```python
from build123d import *

# Parameters (mm, degrees)
SKETCH1_R                = 7.5
SKETCH1_R_2              = 3.15
BOSS_EXTRUDE1_DEPTH      = 13
BOSS_EXTRUDE2_START      = 10
SKETCH2_R                = 7.5
BOSS_EXTRUDE2_DEPTH      = 10
BOSS_EXTRUDE4_DEPTH      = 5
BOSS_EXTRUDE4_DEPTH_BACK = 10
SKETCH7_R                = 4.7
CUT_EXTRUDE2_DEPTH       = 20
SKETCH9_R                = 2.2
CUT_EXTRUDE4_DEPTH       = 37.626493144
CUT_EXTRUDE5_REACH       = 33.329
CUT_EXTRUDE5_END_RADIUS  = 7.5
SKETCH4_R                = 2.5


with BuildPart() as part:
    # Sketch1 → Boss-Extrude1 (new body)
    with BuildSketch(Plane(origin=(0, 0, 0), x_dir=(1, 0, 0), z_dir=(0, 1, 0))):
        with Locations(Location((0, 0, 0), (0, 0, 90))):
            Circle(SKETCH1_R)
        with Locations(Location((0, 0, 0), (0, 0, 90))):
            Circle(SKETCH1_R_2, mode=Mode.SUBTRACT)
    extrude(amount=BOSS_EXTRUDE1_DEPTH)

    # Sketch2 → Boss-Extrude2 (add)
    with BuildSketch(Plane.XZ.offset(BOSS_EXTRUDE2_START)):
        with Locations(Location((0, 0, 0), (0, 0, 270))):
            Circle(SKETCH2_R)
    extrude(amount=-BOSS_EXTRUDE2_DEPTH)

    # Sketch6 → Boss-Extrude4 (add, two sides: drawn at the far end of the back side and taken through both)
    with BuildSketch(Plane(origin=(0, 0, 0), x_dir=(1, 0, 0), z_dir=(0, 1, 0)).offset(-BOSS_EXTRUDE4_DEPTH_BACK)):
        with BuildLine():
            Line((-7.5, 0), (-7.5, 27.5))
            Line((-7.5, 27.5), (7.5, 27.5))
            Line((7.5, 27.5), (7.5, 0))
            ThreePointArc((7.5, 0), (0, 7.5), (-7.5, 0))
        make_face()
    extrude(amount=BOSS_EXTRUDE4_DEPTH + BOSS_EXTRUDE4_DEPTH_BACK)

    # Sketch7 → Cut-Extrude2 (cut)
    with BuildSketch(Plane(origin=(0, 0, -27.5), x_dir=(-1, 0, 0), z_dir=(0, 0, -1))):
        with Locations((0, -2.5)):
            Circle(SKETCH7_R)
    extrude(amount=-CUT_EXTRUDE2_DEPTH, mode=Mode.SUBTRACT)

    # Sketch9 → Cut-Extrude4 (cut, through all)
    with BuildSketch(Plane.XZ.offset(10)):
        with Locations(Location((0, -20.5, 0), (0, 0, 270))):
            Circle(SKETCH9_R)
    extrude(amount=-CUT_EXTRUDE4_DEPTH, mode=Mode.SUBTRACT)

    # Cut-Extrude5: up to this cylinder (the profile starts inside it)
    cut_extrude5_end = Plane(origin=(0, 7.53728, 0), z_dir=(0, -1, 0)) * Cylinder(CUT_EXTRUDE5_END_RADIUS, 82.658, mode=Mode.PRIVATE)
    # Sketch4 → Cut-Extrude5 (cut, up to the surface)
    with BuildSketch(Plane.XY, mode=Mode.PRIVATE) as cut_extrude5_sk1:
        with Locations(Location((0, 7.537279813, 0), (0, 0, 180))):
            Circle(SKETCH4_R)
    cut_extrude5_tool1 = extrude(cut_extrude5_sk1.sketch, amount=CUT_EXTRUDE5_REACH, mode=Mode.PRIVATE) & cut_extrude5_end
    add(cut_extrude5_tool1.solids().sort_by_distance((0, 7.53728, 0))[0], mode=Mode.SUBTRACT)


solid = part.part
```
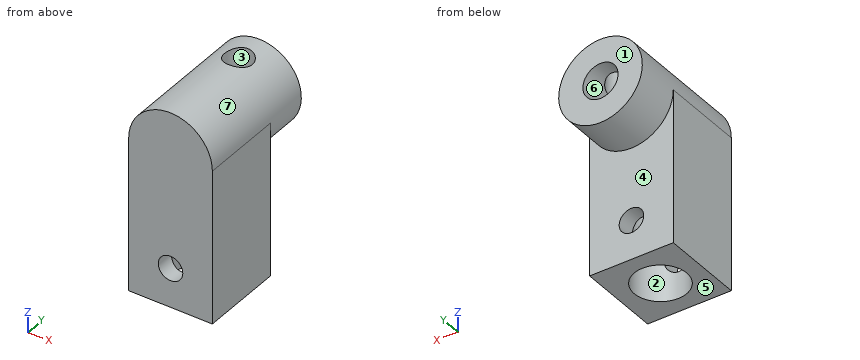
Can you work these out from the model? Positions are in its coordinate system, mm. Face numbers are marked on the shaded views. A direction names the side the tool comes from. Coordinates: 2 decimals unless noted, no trailing zeros. Loops run counter-clockwise (first coordinate to the right, second up) from the corner with the lowest first, then second, coordinate; pieces in that order, holes last. Notation, with made-up numbers: (62, 82.25) - (103, 82.25) arc R18 cw to (103, 106.25) - close; hole circle Ø2 at (82.25, 19). An arc over 180 degrees is marked (long way). Use a Markdown table: item, result.
Item 1: Will these pins go through, and if not, where does the flat tip stop? pin 1 (4 mm diameter, centred on x = 0, z = -20.5, fed in from +Y); pin 2 (3 mm diameter, centred on x = -3.5, y = -5.5, fed in from +Z); pin 3 (6 mm diameter, centred on x = 1.5, z = 1.5, fed in from +Y); pin 4 (4 mm diameter, centred on x = 0, z = 0, fed in from +Y).
Numbers:
| item | result |
|---|---|
| pin 1 | passes through |
| pin 2 | stops at z = 7.23 |
| pin 3 | stops at y = 13 |
| pin 4 | stops at y = 0 |
Item 2: I want a section at A-A on z = -20.5. Please give me the cut outline in (x, y).
Numbers:
| item | result |
|---|---|
| outline | (-7.5, -10) - (-2.2, -10) - (-2.2, -6.65) arc R4.7 cw to (-2.2, 1.65) - (-2.2, 5) - (-7.5, 5) - close; (2.2, -10) - (7.5, -10) - (7.5, 5) - (2.2, 5) - (2.2, 1.65) arc R4.7 cw to (2.2, -6.65) - close |
Item 3: I want a section at D-D on z = -13. Please give me the cut outline in (x, y), and give its area (3 significant figures).
Numbers:
| item | result |
|---|---|
| outline | (-7.5, -10) - (7.5, -10) - (7.5, 5) - (-7.5, 5) - close; hole circle Ø9.4 at (0, -2.5) |
| area | 156 mm2 |
Item 4: I want a section at C-C on y = -2.5. Please give me the cut outline in (x, z), and give its area (3 significant figures).
Numbers:
| item | result |
|---|---|
| outline | (-7.5, -27.5) - (-4.7, -27.5) - (-4.7, -7.5) - (4.7, -7.5) - (4.7, -27.5) - (7.5, -27.5) - (7.5, 0) arc R7.5 ccw to (-7.5, 0) - close |
| area | 313 mm2 |
Item 5: We'd pull the mould along Z, two halves only. Please class the marked faces 4, 5, 6 and 7: released by +Z, released by -Z, zero draft, split by the parting line, or undercut.
Numbers:
| item | result |
|---|---|
| face 4 | zero draft |
| face 5 | released by -Z |
| face 6 | undercut |
| face 7 | split by the parting line |
Item 6: I want a section at B-B on x = 0. Please give me the cut outline in (y, z).
Numbers:
| item | result |
|---|---|
| outline | (-10, -27.5) - (-7.2, -27.5) - (-7.2, -22.7) - (-10, -22.7) - close; (-10, -18.3) - (-7.2, -18.3) - (-7.2, -7.5) - (2.2, -7.5) - (2.2, -18.3) - (5, -18.3) - (5, -7.5) - (13, -7.5) - (13, -3.15) - (0, -3.15) - (0, 3.15) - (5.04, 3.15) - (5.04, 7.5) - (-10, 7.5) - close; (2.2, -27.5) - (5, -27.5) - (5, -22.7) - (2.2, -22.7) - close; (10.04, 3.15) - (13, 3.15) - (13, 7.5) - (10.04, 7.5) - close |
Item 7: For the marked faces 1, 2 and 3, which set-ups out of +Z, -Z, +X, -X, +Y, -Y let a thin tool reach every point of the face, with its end or its side?
Numbers:
| item | result |
|---|---|
| face 1 | +Z, -Z, +X, -X, +Y |
| face 2 | -Z |
| face 3 | +Z |
Item 8: If I drill on probe 1 along X at (y, z) = (-7.8, -20.5); probe 2 along Y at (x, z) = (0, 6.5); probe 3 along X at (y, z) = (-2.75, -17), over which ranges is the centre line in solid material (lowest first)? Write a range as from..to.
Numbers:
| item | result |
|---|---|
| probe 1 | x = -7.5..-2.2, 2.2..7.5 |
| probe 2 | y = -10..5.04, 10.04..13 |
| probe 3 | x = -7.5..-4.69, 4.69..7.5 |
